from build123d import *

# Parameters (mm, degrees)
SKETCH_1_R      = 1.5
EXTRUDE_1_DEPTH = 2
FILLET_1_R      = 1


with BuildPart() as part:
    # 草图1 → 凸台-拉伸1 (new body)
    with BuildSketch(Plane.XY):
        Polygon((160, 46.5), (70.5, 46.5), (70.5, 50.8), (59.5, 50.8), (59.5, 46.5), (-30, 46.5), (-30, -13.5), (160, -13.5), align=None)
        with Locations((-25, 41.5)):
            Circle(SKETCH_1_R, mode=Mode.SUBTRACT)
        with Locations((155, 41.5)):
            Circle(SKETCH_1_R, mode=Mode.SUBTRACT)
        with Locations((-25, -8.5)):
            Circle(SKETCH_1_R, mode=Mode.SUBTRACT)
        with Locations((155, -8.5)):
            Circle(SKETCH_1_R, mode=Mode.SUBTRACT)
    extrude(amount=EXTRUDE_1_DEPTH)

    # 圆角1
    fillet_1_edges = [part.edges().sort_by_distance(p)[0] for p in [
        (59.5, 46.5, 1),
        (59.5, 50.8, 1),
        (70.5, 50.8, 1),
        (70.5, 46.5, 1),
        (160, 46.5, 1),
        (160, -13.5, 1),
        (-30, -13.5, 1),
        (-30, 46.5, 1),
    ]]
    fillet(fillet_1_edges, radius=FILLET_1_R)


solid = part.part
Source: CAD feature listing. Evaluate the final solid. Frame: model axes, mm. Give positions to 0.01 mm unless a question says otherwise; leave off trailing zeros. Write each loop counter-clockwise with the first axis right and the second up, starting at its lowest first coordinate (ties: lowest second). Pieces come first, ordered by that corner, then holes. Notation, with made-up numbers: M 60.5,54 L 110.5,54 A25 cw 110.5,79 Z; hole C 82.5,72.25 d7. An arc over 180 degrees is marked long. Return JSON: item names as keys, results as strings. Group by question number.
1) Pin query (flat end, axial travel): P1, Ø0.6, axis at y = 48.5, z = 0.5, coming from the +X side; P2, Ø1, axis at x = 98.5, z = 1, coming from the +Y side. Return the tip coordinate at first contact, or that it passes through.
2) Cut plane B-B, the plane x = 124. Output: boundary loops of the cut face in (y, z).
3) Cut plane A-A, the plane z = 1.2. Output: boundary loops of the cut face in (x, y).
4) Material intervals for line 1 along Y through (x, z) = (-25, 0.75); line 2 along Y through (x, z) = (3, 0.7), sorted ascending. Write a range as [from, to].
Recorded:
{
 "1": {"P1": "stops at x = 70.5", "P2": "stops at y = 46.5"},
 "2": {"outline": "M -13.5,0 L 46.5,0 L 46.5,2 L -13.5,2 Z"},
 "3": {"outline": "M -30,-12.5 A1 ccw -29,-13.5 L 159,-13.5 A1 ccw 160,-12.5 L 160,45.5 A1 ccw 159,46.5 L 71.5,46.5 A1 cw 70.5,47.5 L 70.5,49.8 A1 ccw 69.5,50.8 L 60.5,50.8 A1 ccw 59.5,49.8 L 59.5,47.5 A1 cw 58.5,46.5 L -29,46.5 A1 ccw -30,45.5 Z; hole C -25,-8.5 d3; hole C -25,41.5 d3; hole C 155,-8.5 d3; hole C 155,41.5 d3"},
 "4": {"line 1": "y = [-13.5, -10], [-7, 40], [43, 46.5]", "line 2": "y = [-13.5, 46.5]"}
}
